The model under review builds one solid part; all positions refer to its coordinate system, in mm. A direction names the side the tool comes from. Give positions to 0.01 mm unless a question says otherwise; leave off trailing zeros. Order: outer loops, then holes, each group sorted by start corner. A loop starts at its lowest first (then second) coordinate and runs counter-clockwise, first axis right, second up.
```python
from build123d import *

# Parameters (mm, degrees)
EXTRUDE_1_DEPTH = 3


with BuildPart() as part:
    # 草图1 → 凸台-拉伸1 (new body)
    with BuildSketch(Plane(origin=(0, 0, 0), x_dir=(1, 0, 0), z_dir=(0, 1, 0))):
        Polygon((25, -8), (25, 0), (23.098111609, 0), (15.799055804, 0), (15.799055804, -4), (14.549055804, -4), (14.549055804, -5), (11.549055804, -5), (11.549055804, -4), (10.299055804, -4), (10.299055804, 0), (3, 0), (0, 0), (0, -8), align=None)
        Polygon((25, -16), (25, -8), (0, -8), (0, -16), (3, -16), (10.299055804, -16), (10.299055804, -12), (11.549055804, -12), (11.549055804, -11), (14.549055804, -11), (14.549055804, -12), (15.799055804, -12), (15.799055804, -16), (23.098111609, -16), align=None)
        Polygon((23.098111609, -19), (23.098111609, -16), (15.799055804, -16), (14.549055804, -16), (14.549055804, -19), align=None)
        Polygon((10.299055804, -16), (3, -16), (3, -19), (11.549055804, -19), (11.549055804, -16), align=None)
        Polygon((3, 3), (3, 0), (10.299055804, 0), (11.549055804, 0), (11.549055804, 3), align=None)
        Polygon((15.799055804, 0), (23.098111609, 0), (23.098111609, 3), (14.549055804, 3), (14.549055804, 0), align=None)
        Polygon((27, 3), (27, 0), (34.200944196, 0), (35.450944196, 0), (35.450944196, 3), align=None)
        Polygon((39.700944196, 0), (47, 0), (47, 3), (38.450944196, 3), (38.450944196, 0), align=None)
        Polygon((27, 0), (25, 0), (25, -8), (50, -8), (50, 0), (47, 0), (39.700944196, 0), (39.700944196, -4), (38.450944196, -4), (38.450944196, -5), (35.450944196, -5), (35.450944196, -4), (34.200944196, -4), (34.200944196, 0), align=None)
        Polygon((50, -8), (25, -8), (25, -16), (27, -16), (34.200944196, -16), (34.200944196, -12), (35.450944196, -12), (35.450944196, -11), (38.450944196, -11), (38.450944196, -12), (39.700944196, -12), (39.700944196, -16), (47, -16), (50, -16), align=None)
        Polygon((34.200944196, -16), (27, -16), (27, -19), (35.450944196, -19), (35.450944196, -16), align=None)
        Polygon((47, -19), (47, -16), (39.700944196, -16), (38.450944196, -16), (38.450944196, -19), align=None)
    extrude(amount=EXTRUDE_1_DEPTH)


solid = part.part
```
1. Insertion check: pin 1 (1.1 mm diameter, centred on y = 1, z = 11.5, fed in from -X). The pin has a flat end and moves straight along its axis. Give the tip position at first contact, or say it passes through.
2. Take a section at A-A (z = 17.5). Write out the cut boundary in (x, y).
3. To check wall thickness, follow line 1 (X direction, y = 0.75, z = 3.75); line 2 (X direction, y = 0.7, z = -1.25); line 3 (Z direction, x = 39, y = 2.65). State the ranges of each line that lie inside material, in increasing order.
4. Take a section at B-B (x = 39). Write out the cut boundary in (y, z), and give its area (3 significant figures).
5. For faces 1 (the flat face through (14.549, 1.5, 11.5)), 2 (the flat face through (27, 1, -2)), 3 (the flat face through (39, 1, 16)), 4 (the flat face through (47, 1, -1)), list the 3-axis set-ups (+Z, -Z, +X, -X, +Y, -Y) from which the entire face can be reached by the end or side of a thin tool; tool diameter is ignored.
6. Take a section at D-D (x = 13). Write out the cut boundary in (y, z), and give its area (3 significant figures).
7. Take a section at C-C (z = 2). Write out the cut boundary in (x, y).
Answer:
1. pin 1: stops at x = 0
2. outline: (3, 0) - (11.55, 0) - (11.55, 3) - (3, 3) - close; (14.55, 0) - (23.1, 0) - (23.1, 3) - (14.55, 3) - close; (27, 0) - (35.45, 0) - (35.45, 3) - (27, 3) - close; (38.45, 0) - (47, 0) - (47, 3) - (38.45, 3) - close
3. line 1: x = 0 to 10.3, 15.8 to 34.2, 39.7 to 50
3. line 2: x = 3 to 11.55, 14.55 to 23.1, 27 to 35.45, 38.45 to 47
3. line 3: z = -3 to 0, 4 to 12, 16 to 19
4. outline: (0, -3) - (3, -3) - (3, 0) - (0, 0) - close; (0, 4) - (3, 4) - (3, 12) - (0, 12) - close; (0, 16) - (3, 16) - (3, 19) - (0, 19) - close
4. area: 42.0 mm2
5. face 1: +Z, +Y, -Y
5. face 2: -Z, +Y, -Y
5. face 3: +Y, -Y
5. face 4: -Z, +X, +Y, -Y
6. outline: (0, 5) - (3, 5) - (3, 11) - (0, 11) - close
6. area: 18.0 mm2
7. outline: (0, 0) - (10.3, 0) - (10.3, 3) - (0, 3) - close; (15.8, 0) - (34.2, 0) - (34.2, 3) - (15.8, 3) - close; (39.7, 0) - (50, 0) - (50, 3) - (39.7, 3) - close
